Verification items for the finished model (mm, model axes). Round coordinates to 2 decimals unless told otherwise and drop trailing zeros. Order: outer loops, then holes, each group sorted by start corner. A loop starts at its lowest first (then second) coordinate and runs counter-clockwise, first axis right, second up. Notation, with made-up numbers: (20.5, 17) -> (44.5, 17) arc R12 cw to (44.5, 22) -> close; hole circle Ø2 at (15, 23.5). An arc over 180 degrees is marked (long way). Return JSON: item names as keys, results as strings. Group by question number.
1) Section check C-C on x = -120.5. Enter the section's corners in (y, z).
2) Section check A-A on y = -0.95. Enter the section's corners in (x, z) (1 decimal), plus the area to 3 significant figures.
3) Depth check by flat-ended pin: pin 1 (1.6 mm diameter, centred on y = -2, z = -11, fed in from +X); pin 2 (1.5 mm diameter, centred on y = -4, z = 44, fed in from -X); pin 3 (1.5 mm diameter, centred on x = -51, y = -3, fed in from -Z); pin 4 (8 mm diameter, centred on x = 12, z = 38, fed in from +Y). Enter the tip coordinate at first touch or a pass-through.
4) Section check B-B on z = 36. Enter the section's corners in (x, y).
5) Scan lines: L1, parallel to X at y = -2.35, z = 36; L2, parallel to Z at x = -73, y = -4.2; L3, parallel to X at y = -4.15, z = 46. Record each from-to range of solid material in increasing order.
6) Section check D-D on z = 70. Enter the section's corners in (x, y).
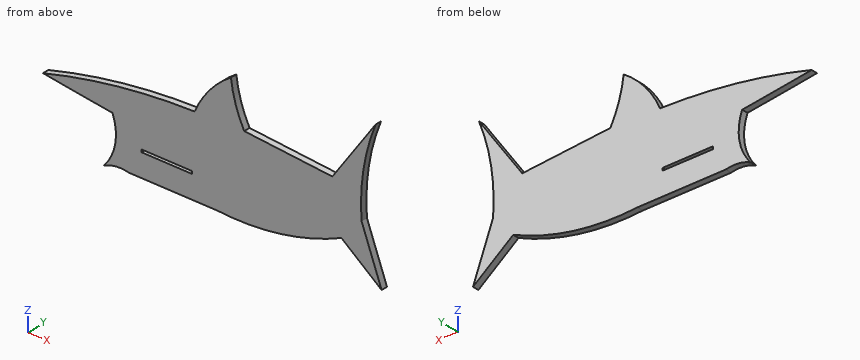
```python
from build123d import *

# Parameters (mm, degrees)
F0_W     = 40
F0_H     = 2
F1_DEPTH = 5


with BuildPart() as f1:
    # F0 (on Front) → F1 (new body)
    with BuildSketch(Plane.XZ):
        with BuildLine():
            Line((64.111737, 27.99553), (-5.684315, 33.335119))
            ThreePointArc((-5.684315, 33.335119), (-12.51556, 49.531418), (-16.191208, 66.720822))
            ThreePointArc((-16.191208, 66.720822), (-33.109228, 51.528336), (-44.980059, 32.134667))
            ThreePointArc((-44.980059, 32.134667), (-105.571318, 26.711963), (-164.980059, 13.6235))
            ThreePointArc((-164.980059, 13.6235), (-137.491015, 10.068821), (-109.980059, 6.687917))
            ThreePointArc((-109.980059, 6.687917), (-107.784091, -14.004458), (-116.903277, -32.70839))
            ThreePointArc((-116.903277, -32.70839), (-107.223293, -29.61905), (-97.073786, -30.102378))
            Line((-97.073786, -30.102378), (-27.073786, -30.102378))
            ThreePointArc((-27.073786, -30.102378), (23.272059, -27.46882), (71.299644, -12.139407))
            Line((71.299644, -12.139407), (103.101424, -36.401451))
            Line((103.101424, -36.401451), (87.200534, 5.6956))
            ThreePointArc((87.200534, 5.6956), (88.69059, 42.109352), (98.391595, 77.238715))
            Line((98.391595, 77.238715), (64.111737, 27.99553))
        make_face()
        with Locations((-67.080881, -11.102378)):
            Rectangle(F0_W, F0_H, mode=Mode.SUBTRACT)
    extrude(amount=F1_DEPTH)


solid = f1.part
```
Check result:
{
 "1": {"outline": "(-5, 7.96) -> (0, 7.96) -> (0, 24.17) -> (-5, 24.17) -> close"},
 "2": {"outline": "(-165, 13.6) arc R4386.4 ccw to (-110, 6.7) arc R37.7 cw to (-116.9, -32.7) arc R28.7 cw to (-97.1, -30.1) -> (-27.1, -30.1) arc R196.9 ccw to (71.3, -12.1) -> (103.1, -36.4) -> (87.2, 5.7) arc R159.8 cw to (98.4, 77.2) -> (64.1, 28) -> (-5.7, 33.3) arc R93.4 cw to (-16.2, 66.7) arc R78.7 ccw to (-45, 32.1) arc R477.1 ccw to start; hole (-87.1, -12.1) -> (-47.1, -12.1) -> (-47.1, -10.1) -> (-87.1, -10.1) -> close", "area": "13,200 mm^2"},
 "3": {"pin 1": "x = 93.81", "pin 2": "x = -39.13", "pin 3": "z = -30.1", "pin 4": "through"},
 "4": {"outline": "(-43.2, -5) -> (-7.06, -5) -> (-7.06, 0) -> (-43.2, 0) -> close; (69.68, -5) -> (87.86, -5) -> (87.86, 0) -> (69.68, 0) -> close"},
 "5": {"L1": "-43.2 to -7.06, 69.68 to 87.86", "L2": "-30.1 to -12.1, -10.1 to 30.6", "L3": "-37.31 to -11.33, 76.65 to 89.35"},
 "6": {"outline": "(93.35, -5) -> (95.67, -5) -> (95.67, 0) -> (93.35, 0) -> close"}
}
